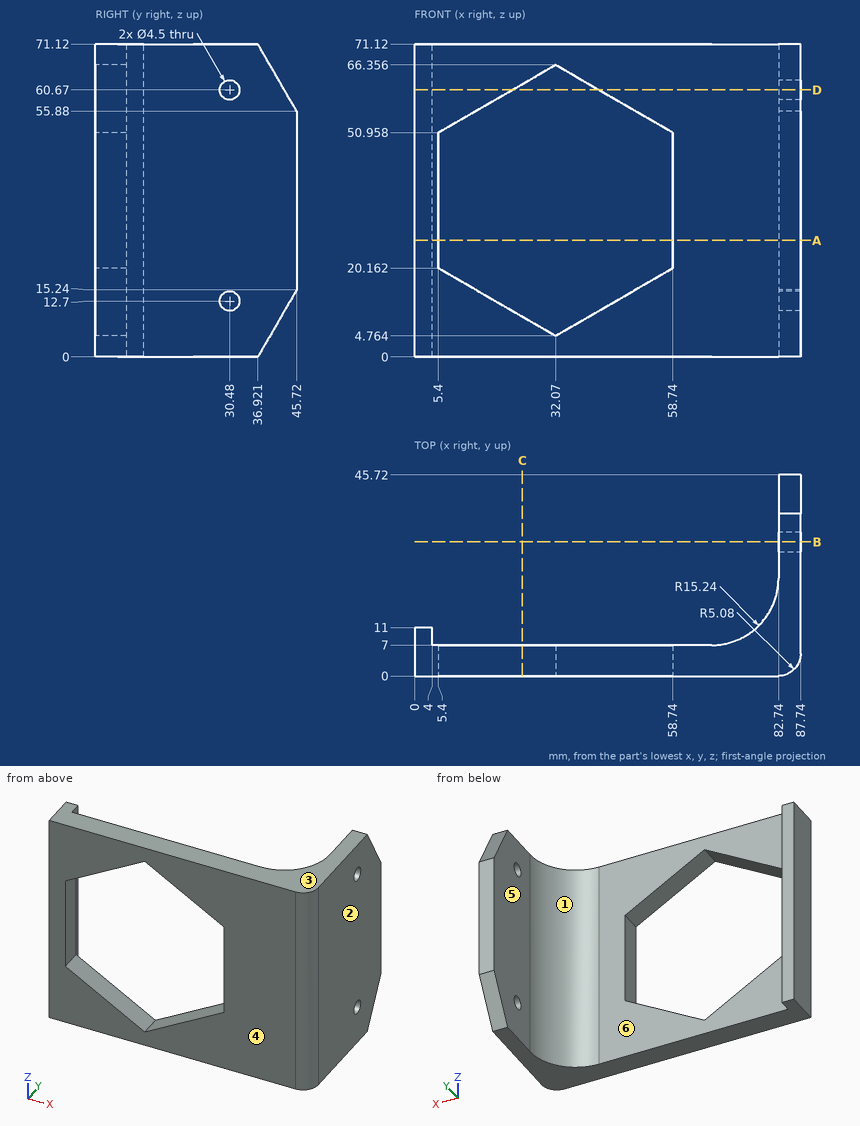
Design review of the part shown in the three views and the two pictorial views. Dimensions are in mm from the part's minimum x, y and z. A direction names the side the tool comes from. Give positions to 0.01 mm unless a question says otherwise; leave off trailing zeros. Write each loop counter-clockwise with the first axis right and the second up, starting at its lowest first coordinate (ties: lowest second). Pieces come first, ordered by that corner, then holes. Notation, with made-up numbers: M 6,-20 L 33,-20 A31 cw 33,8 Z; hole C 6,54.25 d5. An arc over 180 degrees is marked long. One line per question, with ' | ' between items. Start each with the question number.
Item 1: For the marked faces 4, 5 and 6, list the 3-axis set-ups (+Z, -Z, +X, -X, +Y, -Y) from which the entire face can be reached by the end or side of a thin tool; tool diameter is ignored.
Item 2: We need section A-A on z = 26.5. Write out the cut boundary in (x, y), plus the area to 3 significant figures.
Item 3: Draft analysis for pull direction X (two halves, no side actions). For the marked faces 1, 2 and 3, state which applies: released by +X, released by -X, zero draft, split by the parting line, or undercut.
Item 4: We need section B-B on y = 30.48. Write out the cut boundary in (x, z), plus the area to 3 significant figures.
Item 5: We need section D-D on z = 60.67. Write out the cut boundary in (x, y).
Item 6: For pin 1 (2 mm diameter, centred on y = 2, z = 30.5, fed in from +X) (1 decimal); pin 2 (19 mm diameter, centred on y = 30, z = 51.5, fed in from -X); pin 3 (4 mm diameter, centred on y = 32.5, z = 49.5, fed in from -X); pin 4 (5.5 mm diameter, centred on y = 2, z = 34.5, fed in from -X), all flat-tipped, find the tip position at first contact; note any pin that passes through.
Item 7: Wall thickness on line 1 (Z direction, x = 85.7, y = 30.48); line 2 (Z direction, x = 85, y = 30); line 3 (X direction, y = 25, z = 57.5): over which ranges is each line inside the solid? List them lowest first. Write a range as from..to.
Item 8: We need section C-C on x = 24.5. Write out the cut boundary in (y, z) (1 decimal).
Results found:
1) face 4: +Z, -Z, +X, -X, -Y | face 5: +Z, -Z, -X, +Y | face 6: +Z, -Z, +Y
2) outline: M 0,0 L 5.4,0 L 5.4,7 L 4,7 L 4,11 L 0,11 Z; M 58.74,0 L 82.66,0 A5.08 ccw 87.74,5.08 L 87.74,45.72 L 82.74,45.72 L 82.74,22.24 A15.24 cw 67.5,7 L 58.74,7 Z | area: 495 mm2
3) face 1: undercut | face 2: released by +X | face 3: zero draft
4) outline: M 82.74,0 L 87.74,0 L 87.74,10.45 L 82.74,10.45 Z; M 82.74,14.95 L 87.74,14.95 L 87.74,58.42 L 82.74,58.42 Z; M 82.74,62.92 L 87.74,62.92 L 87.74,71.12 L 82.74,71.12 Z | area: 311 mm2
5) outline: M 0,0 L 22.22,0 L 22.22,7 L 4,7 L 4,11 L 0,11 Z; M 41.92,0 L 82.66,0 A5.08 ccw 87.74,5.08 L 87.74,28.23 L 82.74,28.23 L 82.74,22.24 A15.24 cw 67.5,7 L 41.92,7 Z; M 82.74,32.73 L 87.74,32.73 L 87.74,42.95 L 82.74,42.95 Z
6) pin 1: stops at x = 87.3 | pin 2: stops at x = 82.64 | pin 3: stops at x = 82.74 | pin 4: stops at x = 0
7) line 1: z = 0..10.45, 14.95..58.42, 62.92..71.12 | line 2: z = 0..10.5, 14.9..58.47, 62.87..71.12 | line 3: x = 82.74..87.74
8) outline: M 0,0 L 7,0 L 7,9.1 L 0,9.1 Z; M 0,62 L 7,62 L 7,71.1 L 0,71.1 Z
